Model file for the job. Use its own axes, mm. A direction names the side the tool comes from. Coordinates: 2 decimals unless noted, no trailing zeros. Order: outer loops, then holes, each group sorted by start corner. A loop starts at its lowest first (then second) coordinate and runs counter-clockwise, first axis right, second up.
Autodesk Inventor part; units mm, degrees
ref_plane "YZ Plane" through (0, 0, 0) normal (1, 0, 0) x (0, 1, 0)
ref_plane "XZ Plane" through (0, 0, 0) normal (0, 1, 0) x (-1, 0, 0)
ref_plane "XY Plane" through (0, 0, 0) normal (0, 0, 1) x (1, 0, 0)
sketch "Esquisse1" plane through (0, 0, 0) normal (0, 0, 1) x (1, 0, 0)
  circle A0 centre (0, -2.0906) radius 7
  point P0 (0, 0)
  dimension "d0" = 14
extrude "Extrusion1" add sketch "Esquisse1" along normal blind 2
sketch "Esquisse2" plane through (0, -2.0906, 2) normal (0, 0, 1) x (1, 0, 0)
  circle A0 centre (0, 0) radius 2.1
  circle A1 centre (0, 0) radius 2.5
  point P0 (0, 2.0906)
  dimension "d3" = 4.2
  dimension "d4" = 5
extrude "Extrusion2" add sketch "Esquisse2" along normal blind 4
properties part number "ajust_plaque"
Q1. Cut at A-A, the plane x = 0. List the corners of the cut face in (y, z), plus the area to 3 significant figures.
Established:
outline: (-9.09, 0) - (4.91, 0) - (4.91, 2) - (0.41, 2) - (0.41, 6) - (0.01, 6) - (0.01, 2) - (-4.19, 2) - (-4.19, 6) - (-4.59, 6) - (-4.59, 2) - (-9.09, 2) - close
area: 31.2 mm2
Q2. Probe line 1 (Y direction, x = 0, z = 5.1); line 2 (X direction, y = -2, z = 2.6); line 3 (Z direction, x = 0.25, y = -5.5). List the from-to ranges inside material, lowest first.
Established:
line 1: y = -4.59 to -4.19, 0.01 to 0.41
line 2: x = -2.5 to -2.1, 2.1 to 2.5
line 3: z = 0 to 2
Q3. Cut at D-D, the plane y = 0.75. List the corners of the cut face in (x, z), plus the area to 3 significant figures.
Established:
outline: (-6.4, 0) - (6.4, 0) - (6.4, 2) - (-6.4, 2) - close
area: 25.6 mm2
Q4. Mould opens along X. For faces 3 (the face through (-0.46, -0.04, 3.97)), 4 (the face through (-1, 0, 6)), 5 (the face through (-0.54, 0.35, 3.97)) say: pulls with the +X half, pulls with the -X half, needs draft (parallel to the pull), parting line crosses it, or undercut.
Established:
face 3: undercut
face 4: needs draft
face 5: parting line crosses it
Q5. Which spindle directions (+Z, -Z, +X, -X, +Y, -Y) get a long thin tool onto all of the face, cutting with end or side? Do faces 1 (the face through (0, -2, 2)), 2 (the face through (0, -2, 0)). Say none if no direction does.
Established:
face 1: +Z
face 2: -Z, +X, -X, +Y, -Y
Q6. Cut at B-B, the plane x = 1.75. List the corners of the cut face in (y, z), plus the area to 3 significant figures.
Established:
outline: (-8.87, 0) - (4.69, 0) - (4.69, 2) - (-0.31, 2) - (-0.31, 6) - (-0.93, 6) - (-0.93, 2) - (-3.25, 2) - (-3.25, 6) - (-3.88, 6) - (-3.88, 2) - (-8.87, 2) - close
area: 32.1 mm2
Q7. Cut at C-C, the plane y = -5.25. List the corners of the cut face in (x, z), plus the area to 3 significant figures.
Established:
outline: (-6.25, 0) - (6.25, 0) - (6.25, 2) - (-6.25, 2) - close
area: 25.0 mm2
Q8. Drop flat-ended pins along their axis: P1, Ø4, axis at x = 2, y = -5, coming from the +Z side; P2, Ø4, axis at x = 0, y = -2.09, coming from the +Z side; P3, Ø1, axis at x = -0.5, z = 3.5, coming from the +Y side; P4, Ø1, axis at y = 1.5, z = 1.5, coming from the -X side. Give the stop position or say it passes through.
Established:
P1: stops at z = 6
P2: stops at z = 2
P3: stops at y = 0.41
P4: stops at x = -6.28
